Source: three-view drawing plus pictorial views. Frame: mm from the lowest corner of the part. Give positions to 0.01 mm unless a question says otherwise; leave off trailing zeros. Write each loop counter-clockwise with the first axis right and the second up, starting at its lowest first coordinate (ties: lowest second). Pieces come first, ordered by that corner, then holes.
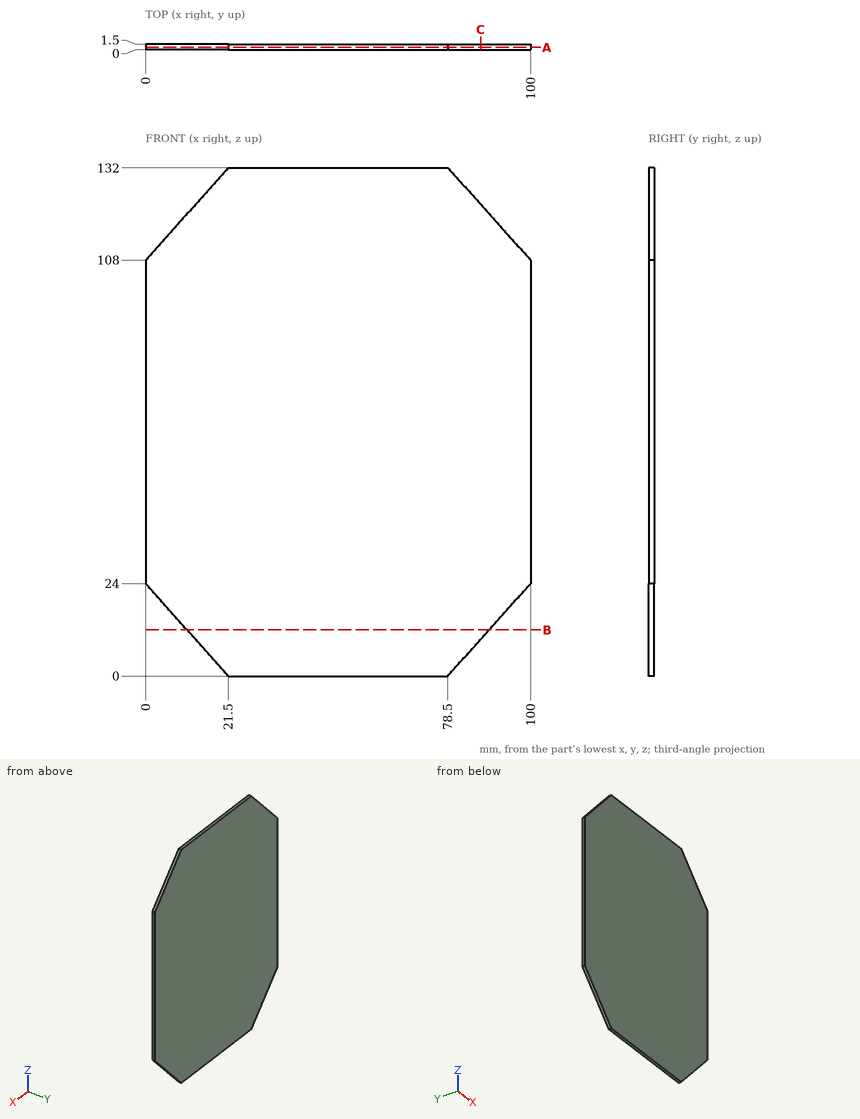
Q1. Ray query, line 1 along Z through (x, y) = (84.5, 0.25); line 2 along Z through (x, y) = (79, 0.75); line 3 along X through (y, z) = (0.5, 115). Return the intervals inside material, ascending.
Filled sheet:
line 1: z = 6.7 to 125.3
line 2: z = 0.56 to 131.44
line 3: x = 6.27 to 93.73
Q2. Section C-C on x = 87. Output: boundary loops of the cut face in (y, z), plus the area to 3 significant figures.
Filled sheet:
outline: (0, 9.49) - (1.5, 9.49) - (1.5, 122.51) - (0, 122.51) - close
area: 170 mm2
Q3. Section B-B on z = 12. Output: boundary loops of the cut face in (x, y), plus the area to 3 significant figures.
Filled sheet:
outline: (10.75, 0) - (89.25, 0) - (89.25, 1.5) - (10.75, 1.5) - close
area: 118 mm2
Q4. Section A-A on y = 0.6. Output: boundary loops of the cut face in (x, z), plus the area to 3 significant figures.
Filled sheet:
outline: (0, 24) - (21.5, 0) - (78.5, 0) - (100, 24) - (100, 108) - (78.5, 132) - (21.5, 132) - (0, 108) - close
area: 12,200 mm2
